from build123d import *

# Parameters (mm, degrees)
SALIENTE_EXTRUIR1_DEPTH      = 5
CROQUIS4_R                   = 3.5
CORTAR_EXTRUIR3_DEPTH        = 15
CROQUIS5_R                   = 1.5
CORTAR_EXTRUIR4_DEPTH        = 10
SALIENTE_EXTRUIR2_DEPTH      = 3
SALIENTE_EXTRUIR2_DEPTH_BACK = 3


with BuildPart() as part:
    # Croquis1 → Saliente-Extruir1 (new, symmetric)
    with BuildSketch(Plane.XY):
        Polygon((3, -8.75), (3, 13.75), (0, 13.75), (0, -13.75), (10, -13.75), (10, -8.75), align=None)
        Polygon((0, -13.75), (0, 13.75), (-3, 13.75), (-3, -8.75), (-10, -8.75), (-10, -13.75), align=None)
    extrude(amount=SALIENTE_EXTRUIR1_DEPTH, both=True)

    # Croquis4 → Cortar-Extruir3 (cut)
    with BuildSketch(Plane(origin=(3, 0, 0), x_dir=(0, 0, -1), z_dir=(1, 0, 0))):
        with Locations(Location((0, 3.55, 0), (0, 0, 90))):
            Circle(CROQUIS4_R)
    extrude(amount=-CORTAR_EXTRUIR3_DEPTH, mode=Mode.SUBTRACT)

    # Croquis5 → Cortar-Extruir4 (cut)
    with BuildSketch(Plane.XZ.offset(13.75)):
        with Locations((-6, 0)):
            Circle(CROQUIS5_R)
        with Locations(Location((6, 0, 0), (0, 0, 180))):
            Circle(CROQUIS5_R)
    extrude(amount=-CORTAR_EXTRUIR4_DEPTH, mode=Mode.SUBTRACT)

    # Croquis6 → Saliente-Extruir2 (add, two sides: drawn at the far end of the back side and taken through both)
    with BuildSketch(Plane(origin=(0, 0, 0), x_dir=(0, 0, -1), z_dir=(1, 0, 0)).offset(-SALIENTE_EXTRUIR2_DEPTH_BACK)):
        with BuildLine():
            ThreePointArc((0.274787705, 7.039196429), (0, 7.05), (-0.274787705, 7.039196429))
            ThreePointArc((-0.274787705, 7.039196429), (0, 6.775), (0.274787705, 7.039196429))
        make_face()
        with BuildLine():
            ThreePointArc((0.994227663, 6.905817539), (0.727690918, 6.973516603), (0.456661795, 7.020080691))
            ThreePointArc((0.456661795, 7.020080691), (0.670515203, 6.704526012), (0.994227663, 6.905817539))
        make_face()
        with BuildLine():
            ThreePointArc((1.670215102, 6.625773319), (1.423578251, 6.747409102), (1.168152983, 6.849305777))
            ThreePointArc((1.168152983, 6.849305777), (1.311725674, 6.496184101), (1.670215102, 6.625773319))
        make_face()
        with BuildLine():
            ThreePointArc((2.273206126, 6.211303047), (2.057248383, 6.38155948), (1.82859028, 6.534335368))
            ThreePointArc((1.82859028, 6.534335368), (1.895607439, 6.159079807), (2.273206126, 6.211303047))
        make_face()
        with BuildLine():
            ThreePointArc((2.776847135, 5.680521061), (2.601006889, 5.891957122), (2.409109407, 6.088935183))
            ThreePointArc((2.409109407, 6.088935183), (2.396642062, 5.707946206), (2.776847135, 5.680521061))
        make_face()
        with BuildLine():
            ThreePointArc((3.159126598, 5.056625081), (3.031088913, 5.3), (2.884338893, 5.532571348))
            ThreePointArc((2.884338893, 5.532571348), (2.792931927, 5.1625), (3.159126598, 5.056625081))
        make_face()
        with BuildLine():
            ThreePointArc((3.403337071, 4.366882356), (3.328697807, 4.63155948), (3.233508929, 4.889559631))
            ThreePointArc((3.233508929, 4.889559631), (3.067157265, 4.546579807), (3.403337071, 4.366882356))
        make_face()
        with BuildLine():
            ThreePointArc((3.498805382, 3.641437951), (3.480826634, 3.915849621), (3.441359109, 4.18800273))
            ThreePointArc((3.441359109, 4.18800273), (3.207333113, 3.887104294), (3.498805382, 3.641437951))
        make_face()
        with BuildLine():
            ThreePointArc((3.441359109, 2.91199727), (3.480826634, 3.184150379), (3.498805382, 3.458562049))
            ThreePointArc((3.498805382, 3.458562049), (3.207333113, 3.212895706), (3.441359109, 2.91199727))
        make_face()
        with BuildLine():
            ThreePointArc((3.233508929, 2.210440369), (3.328697807, 2.46844052), (3.403337071, 2.733117644))
            ThreePointArc((3.403337071, 2.733117644), (3.067157265, 2.553420193), (3.233508929, 2.210440369))
        make_face()
        with BuildLine():
            ThreePointArc((2.884338893, 1.567428652), (3.031088913, 1.8), (3.159126598, 2.043374919))
            ThreePointArc((3.159126598, 2.043374919), (2.792931927, 1.9375), (2.884338893, 1.567428652))
        make_face()
        with BuildLine():
            ThreePointArc((2.409109407, 1.011064817), (2.601006889, 1.208042878), (2.776847135, 1.419478939))
            ThreePointArc((2.776847135, 1.419478939), (2.396642062, 1.392053794), (2.409109407, 1.011064817))
        make_face()
        with BuildLine():
            ThreePointArc((1.82859028, 0.565664632), (2.057248383, 0.71844052), (2.273206126, 0.888696953))
            ThreePointArc((2.273206126, 0.888696953), (1.895607439, 0.940920193), (1.82859028, 0.565664632))
        make_face()
        with BuildLine():
            ThreePointArc((1.168152983, 0.250694223), (1.423578251, 0.352590898), (1.670215102, 0.474226681))
            ThreePointArc((1.670215102, 0.474226681), (1.311725674, 0.603815899), (1.168152983, 0.250694223))
        make_face()
        with BuildLine():
            ThreePointArc((0.456661795, 0.079919309), (0.727690918, 0.126483397), (0.994227663, 0.194182461))
            ThreePointArc((0.994227663, 0.194182461), (0.670515203, 0.395473988), (0.456661795, 0.079919309))
        make_face()
        with BuildLine():
            ThreePointArc((-0.274787705, 0.060803571), (0, 0.05), (0.274787705, 0.060803571))
            ThreePointArc((0.274787705, 0.060803571), (0, 0.325), (-0.274787705, 0.060803571))
        make_face()
        with BuildLine():
            ThreePointArc((-0.994227663, 0.194182461), (-0.727690918, 0.126483397), (-0.456661795, 0.079919309))
            ThreePointArc((-0.456661795, 0.079919309), (-0.670515203, 0.395473988), (-0.994227663, 0.194182461))
        make_face()
        with BuildLine():
            ThreePointArc((-1.670215102, 0.474226681), (-1.423578251, 0.352590898), (-1.168152983, 0.250694223))
            ThreePointArc((-1.168152983, 0.250694223), (-1.311725674, 0.603815899), (-1.670215102, 0.474226681))
        make_face()
        with BuildLine():
            ThreePointArc((-2.273206126, 0.888696953), (-2.057248383, 0.71844052), (-1.82859028, 0.565664632))
            ThreePointArc((-1.82859028, 0.565664632), (-1.895607439, 0.940920193), (-2.273206126, 0.888696953))
        make_face()
        with BuildLine():
            ThreePointArc((-2.776847135, 1.419478939), (-2.601006889, 1.208042878), (-2.409109407, 1.011064817))
            ThreePointArc((-2.409109407, 1.011064817), (-2.396642062, 1.392053794), (-2.776847135, 1.419478939))
        make_face()
        with BuildLine():
            ThreePointArc((-3.159126598, 2.043374919), (-3.031088913, 1.8), (-2.884338893, 1.567428652))
            ThreePointArc((-2.884338893, 1.567428652), (-2.792931927, 1.9375), (-3.159126598, 2.043374919))
        make_face()
        with BuildLine():
            ThreePointArc((-3.403337071, 2.733117644), (-3.328697807, 2.46844052), (-3.233508929, 2.210440369))
            ThreePointArc((-3.233508929, 2.210440369), (-3.067157265, 2.553420193), (-3.403337071, 2.733117644))
        make_face()
        with BuildLine():
            ThreePointArc((-3.498805382, 3.458562049), (-3.480826634, 3.184150379), (-3.441359109, 2.91199727))
            ThreePointArc((-3.441359109, 2.91199727), (-3.207333113, 3.212895706), (-3.498805382, 3.458562049))
        make_face()
        with BuildLine():
            ThreePointArc((-3.441359109, 4.18800273), (-3.480826634, 3.915849621), (-3.498805382, 3.641437951))
            ThreePointArc((-3.498805382, 3.641437951), (-3.207333113, 3.887104294), (-3.441359109, 4.18800273))
        make_face()
        with BuildLine():
            ThreePointArc((-3.233508929, 4.889559631), (-3.328697807, 4.63155948), (-3.403337071, 4.366882356))
            ThreePointArc((-3.403337071, 4.366882356), (-3.067157265, 4.546579807), (-3.233508929, 4.889559631))
        make_face()
        with BuildLine():
            ThreePointArc((-2.884338893, 5.532571348), (-3.031088913, 5.3), (-3.159126598, 5.056625081))
            ThreePointArc((-3.159126598, 5.056625081), (-2.792931927, 5.1625), (-2.884338893, 5.532571348))
        make_face()
        with BuildLine():
            ThreePointArc((-2.409109407, 6.088935183), (-2.601006889, 5.891957122), (-2.776847135, 5.680521061))
            ThreePointArc((-2.776847135, 5.680521061), (-2.396642062, 5.707946206), (-2.409109407, 6.088935183))
        make_face()
        with BuildLine():
            ThreePointArc((-1.82859028, 6.534335368), (-2.057248383, 6.38155948), (-2.273206126, 6.211303047))
            ThreePointArc((-2.273206126, 6.211303047), (-1.895607439, 6.159079807), (-1.82859028, 6.534335368))
        make_face()
        with BuildLine():
            ThreePointArc((-1.168152983, 6.849305777), (-1.423578251, 6.747409102), (-1.670215102, 6.625773319))
            ThreePointArc((-1.670215102, 6.625773319), (-1.311725674, 6.496184101), (-1.168152983, 6.849305777))
        make_face()
        with BuildLine():
            ThreePointArc((-0.456661795, 7.020080691), (-0.727690918, 6.973516603), (-0.994227663, 6.905817539))
            ThreePointArc((-0.994227663, 6.905817539), (-0.670515203, 6.704526012), (-0.456661795, 7.020080691))
        make_face()
    extrude(amount=SALIENTE_EXTRUIR2_DEPTH + SALIENTE_EXTRUIR2_DEPTH_BACK)


solid = part.part
Part model, mm, in its own coordinate system. A direction names the side the tool comes from. Coordinates: 2 decimals unless noted, no trailing zeros. Loops run counter-clockwise (first coordinate to the right, second up) from the corner with the lowest first, then second, coordinate; pieces in that order, holes last. Notation, with made-up numbers: (75, 35.25) -> (112, 35.25) arc R4 ccw to (112, 40.25) -> close; hole circle Ø2 at (-5.5, -39). An arc over 180 degrees is marked (long way). Use a Markdown table: item, result. Add a question column.
Item 1: Pull direction X, two halves, no side cores. Call faces 4 (the flat face through (-10, -11, 0)), 5 (the flat face through (-7.2, -8.75, 1.2)), 6 (the cylindrical face through (7.5, -11.28, -0.07)): +X half, -X half, draft (parallel to the pull), parting line (faces both ways), or undercut.
Item 2: Probe probe 1 along Z at (x, y) = (6, -11.9); probe 2 along X at (y, z) = (8, 0); probe 3 along Y at (x, z) = (-5.75, 3.5). List the from-to ranges inside material, lowest first.
Item 3: Flat gauge pins, fed straight in: P1, Ø2, axis at x = -8, z = 2.5, coming from the +Y side; P2, Ø1.8, axis at x = 6, z = 0, coming from the +Y side; P3, Ø5, axis at y = 1, z = -2, coming from the -X side; P4, Ø5, axis at y = 6.5, z = -1.5, coming from the +X side. Where does each tip first touch, or does it go through?
Item 4: Band-saw the part on B-B on y = -2. Write the cut outline in (x, z).
Item 5: Band-saw the part on C-C on x = 3.5. Write the cut outline in (y, z).
Item 6: Which spindle directions (+Z, -Z, +X, -X, +Y, -Y) get a long thin tool onto all of the face, cutting with end or side? Do faces 1 (the flat face through (-3, 0, 0)), 2 (the flat face through (0, -3, 5)), 3 (the flat face through (7.3, -8.75, 1.2)). Say none if no direction does.
Item 7: Band-saw the part on A-A on x = 6.5. Write the cut outline in (y, z), plus the area to 3 significant figures.
Geometry says:
| question | item | result |
|---|---|---|
| 1 | face 4 | -X half |
| 1 | face 5 | draft |
| 1 | face 6 | undercut |
| 2 | probe 1 | -5 to -1.5, 1.5 to 5 |
| 2 | probe 2 | -3 to 3 |
| 2 | probe 3 | -13.75 to -8.75 |
| 3 | P1 | y = -8.75 |
| 3 | P2 | through |
| 3 | P3 | x = -3 |
| 3 | P4 | x = 3 |
| 4 | outline | (-3, -5) -> (3, -5) -> (3, 5) -> (-3, 5) -> close |
| 5 | outline | (-13.75, -5) -> (-8.75, -5) -> (-8.75, 5) -> (-13.75, 5) -> close |
| 6 | face 1 | +Z, -Z, -X, +Y |
| 6 | face 2 | +Z, +X, -X, +Y, -Y |
| 6 | face 3 | +Z, -Z, +X, +Y |
| 7 | outline | (-13.75, -5) -> (-8.75, -5) -> (-8.75, -1.41) -> (-13.75, -1.41) -> close; (-13.75, 1.41) -> (-8.75, 1.41) -> (-8.75, 5) -> (-13.75, 5) -> close |
| 7 | area | 35.9 mm² |
